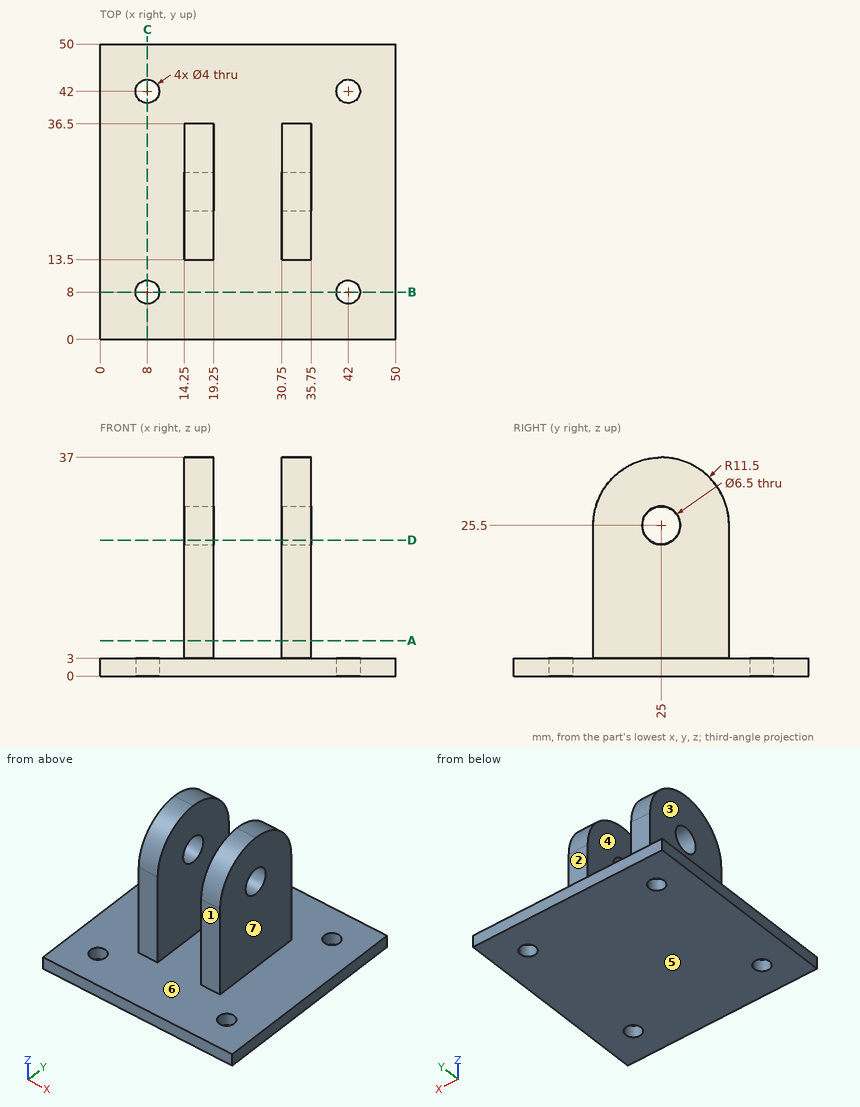
Geometry: see drawing. Coordinates: mm, zero at the bounding-box minimum. A direction names the side the tool comes from. Coordinates: 2 decimals unless noted, no trailing zeros. Order: outer loops, then holes, each group sorted by start corner. A loop starts at its lowest first (then second) coordinate and runs counter-clockwise, first axis right, second up. Notation, with made-up numbers: (-4.75, 42) - (3.25, 42) arc R8 cw to (3.25, 49) - close; hole circle Ø5 at (32.5, 48.5). An arc over 180 degrees is marked (long way). Write each question's results on one line, items separated by ' | '.
1) Pull-direction query (X, two-part tool) for the marked faces 4, 5, 6 and 7; classes: pulls with the +X half, pulls with the -X half, needs draft (parallel to the pull), parting line crosses it, or undercut.
Results list:
face 4: undercut | face 5: needs draft | face 6: undercut | face 7: pulls with the +X half
2) Section B-B, the plane y = 8. Return loops of the section in (x, z).
Results list:
outline: (0, 0) - (6, 0) - (6, 3) - (0, 3) - close; (10, 0) - (40, 0) - (40, 3) - (10, 3) - close; (44, 0) - (50, 0) - (50, 3) - (44, 3) - close
3) Section D-D, the plane z = 23. Return loops of the section in (x, y).
Results list:
outline: (14.25, 13.5) - (19.25, 13.5) - (19.25, 22.92) - (14.25, 22.92) - close; (14.25, 27.08) - (19.25, 27.08) - (19.25, 36.5) - (14.25, 36.5) - close; (30.75, 13.5) - (35.75, 13.5) - (35.75, 22.92) - (30.75, 22.92) - close; (30.75, 27.08) - (35.75, 27.08) - (35.75, 36.5) - (30.75, 36.5) - close
4) Section A-A, the plane z = 6. Return loops of the section in (x, y), plus the area to 3 significant figures.
Results list:
outline: (14.25, 13.5) - (19.25, 13.5) - (19.25, 36.5) - (14.25, 36.5) - close; (30.75, 13.5) - (35.75, 13.5) - (35.75, 36.5) - (30.75, 36.5) - close | area: 230 mm^2
5) Pin query (flat end, axial travel): pin 1 (7 mm diameter, centred on y = 30, z = 13, fed in from +X); pin 2 (5.5 mm diameter, centred on x = 32.5, z = 12, fed in from -Y); pin 3 (3 mm diameter, centred on x = 42, y = 8, fed in from +Z); pin 4 (8 mm diameter, centred on x = 43, y = 39, fed in from +Z). Return the tip coordinate at first contact, or that it passes through.
Results list:
pin 1: x = 35.75 | pin 2: y = 13.5 | pin 3: through | pin 4: z = 3
6) Line query: line 1 (Y direction, x = 8, z = 2); line 2 (Z direction, x = 17.3, y = 25); line 3 (Z direction, x = 17, y = 23) (1 decimal). Output: solid intervals per line, ascending. Write a range as from..to.
Results list:
line 1: 0..6, 10..40, 44..50 | line 2: 0..22.25, 28.75..37 | line 3: 0..22.9, 28.1..36.8
7) Set-up query: the marked faces 1, 2 and 3. Return all of +Z, -Z, +X, -X, +Y, -Y with unobstructed straight access to the full face (end or side cutting, diameter ignored); none if empty.
Results list:
face 1: +Z, +X, -X, -Y | face 2: +Z, +X, -X, +Y | face 3: +Z, -X, +Y, -Y
